Design review of the part built by this model. Coordinates are the model's own, in mm. Face numbers are marked on the shaded views. Round coordinates to 2 decimals unless told otherwise and drop trailing zeros. Loops run counter-clockwise (first coordinate to the right, second up) from the corner with the lowest first, then second, coordinate; pieces in that order, holes last. Notation, with made-up numbers: (63.25, 19) - (105.25, 19) arc R24 ccw to (105.25, 32) - close; hole circle Ø9 at (59.25, 88). An arc over 180 degrees is marked (long way). Return JSON: item names as keys, results as strings. Group by question number.
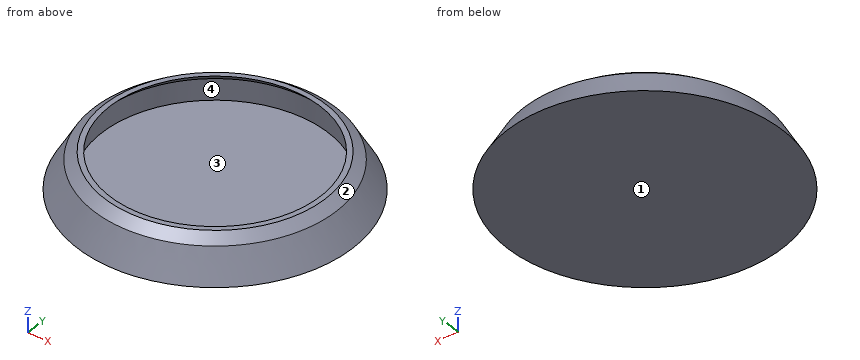
from build123d import *

# Parameters (mm, degrees)
F0_R     = 23
F1_DEPTH = 5.5
F2_T     = -1.5


with BuildPart() as f1:
    # F0 (on Top) → F1 (new body)
    with BuildSketch(Plane.XY):
        Circle(F0_R)
    extrude(amount=F1_DEPTH)

    # F2
    f2_openings = [f1.faces().sort_by_distance(p)[0] for p in [
        (0, 0, 5.5),
    ]]
    offset(amount=F2_T, openings=f2_openings)

    # F3 (on Front) → F4 (revolve)
    with BuildSketch(Plane.XZ):
        Polygon((26.181743, 0), (23, 5.5), (23, 0), align=None)
    revolve(axis=Axis((0, 0, 13.063222), (0, 0, 1)))

    # F5 (on Front) → F6 (revolve)
    with BuildSketch(Plane.XZ):
        Polygon((-21.499641, 5.5), (-20, 7.014853), (-21, 7.014853), (-22.999849, 5.5), align=None)
    revolve(axis=Axis((0, 0, 13.958684), (0, 0, -1)))


solid = f1.part
Q1. Draft analysis for pull direction X (two halves, no side actions). For the marked faces 1, 2, 3 and 4, state which applies: pulls with the +X half, pulls with the -X half, needs draft (parallel to the pull), parting line crosses it, or undercut.
Q2. For line 1 (X direction, y = -18, z = 5.25); line 2 (Z direction, x = 3.5, y = -20.5); line 3 (Z direction, x = 12, y = -5), list the stretches that pass through material, from the lowest coordinate up.
Q3. Insertion check: pin 1 Ø13 at (x, y) = (0, -6.5) entering from +Z; pin 2 Ø3 at (y, z) = (3.5, 3) entering from -X; pin 3 Ø3 at (y, z) = (9, 2) entering from -X. Each pin has a flat end and moves straight along its axis. Give the tip position at first contact, or say it passes through.
Q4. Add section C-C, the plane z = 4.25. State the section outline as (x, y) points.
Evaluation:
{
 "1": {"face 1": "needs draft", "face 2": "parting line crosses it", "face 3": "undercut", "face 4": "undercut"},
 "2": {"line 1": "-14.55 to -11.76, 11.76 to 14.55", "line 2": "0 to 1.5, 6.21 to 7.01", "line 3": "0 to 1.5"},
 "3": {"pin 1": "z = 1.5", "pin 2": "x = -25.09", "pin 3": "x = -24.42"},
 "4": {"outline": "circle Ø47.45 at (0, 0); hole circle Ø43 at (0, 0)"}
}
